The listing builds one solid part. Answer for the finished solid, in the listing's coordinates (mm). Face numbers are marked on the shaded views. Give positions to 0.01 mm unless a question says otherwise; leave off trailing zeros. Order: outer loops, then holes, each group sorted by start corner. A loop starts at its lowest first (then second) coordinate and runs counter-clockwise, first axis right, second up. Notation, with made-up numbers: (22, -17) - (26, -17) arc R24 ccw to (26, -1) - close; hole circle Ø2 at (23.5, 56). An arc over 180 degrees is marked (long way). Answer as a JSON object with one key per item and string values. Group by question number.
Q1. The mould has two halves that part along Y. Classify the marked faces 1 and 2: released by +Y, released by -Y, zero draft, split by the parting line, or undercut.
Q2. Consider line 1 (Y direction, x = 59.5, z = 9.5); line 2 (X direction, y = -17.5, z = 1.25); line 3 (Y direction, x = 11, z = -0.5). Determine where each line is inside the solid, lowest interval first.
Q3. A cutting plane is placed at C-C, the plane y = -31. Give the vertices of the cut face in (x, z), and give its area (3 significant figures).
Q4. Given pin 1 (2 mm diameter, centred on x = 16.5, y = -4, fed in from +Z); pin 2 (12 mm diameter, centred on x = 37, z = 12.5, fed in from +Y); pin 3 (9.5 mm diameter, centred on y = -13, z = 9, fed in from -X); pin 4 (10.5 mm diameter, centred on x = 26, z = 4, fed in from +Y), each flat-ended and moving along its own axis, determine where each tip first touches the part or whether it passes through.
Q5. A cutting plane is placed at A-A, the plane z = -1.25. Give the vertices of the cut face in (x, y), and give its area (3 significant figures).
Q6. A cutting plane is placed at B-B, the plane x = 45.5. Give the vertices of the cut face in (y, z).
from build123d import *

# Parameters (mm, degrees)
SKETCH1_W           = 52
SKETCH1_H           = 32
BOSS_EXTRUDE1_DEPTH = 3
SKETCH2_W           = 4
SKETCH2_H           = 32
BOSS_EXTRUDE2_DEPTH = 20
FILLET1_R           = 3
SKETCH4_R           = 1.725
CUT_EXTRUDE2_DEPTH  = 3
SKETCH6_W           = 20
SKETCH6_H           = 14
CUT_EXTRUDE3_DEPTH  = 3
SKETCH7_W           = 8.2
SKETCH7_H           = 5.8
SKETCH7_W_2         = 5.8
SKETCH7_H_2         = 3.4
BOSS_EXTRUDE4_DEPTH = 6
SKETCH10_R          = 4.9
SKETCH10_R_2        = 4
BOSS_EXTRUDE6_DEPTH = 10
SKETCH8_R           = 5.4
SKETCH8_R_2         = 4.25
BOSS_EXTRUDE5_DEPTH = 6
FILLET2_R           = 2
FILLET3_R           = 3
BOSS_EXTRUDE7_DEPTH = 48


with BuildPart() as part:
    # Sketch1 → Boss-Extrude1 (new body)
    with BuildSketch(Plane.XY):
        with Locations((26, -16)):
            Rectangle(SKETCH1_W, SKETCH1_H)
    extrude(amount=BOSS_EXTRUDE1_DEPTH)

    # Sketch2 → Boss-Extrude2 (add)
    with BuildSketch(Plane(origin=(0, 0, 2), x_dir=(-1, 0, 0), z_dir=(0, 0, -1))):
        with Locations((-50, -16)):
            Rectangle(SKETCH2_W, SKETCH2_H)
    extrude(amount=-BOSS_EXTRUDE2_DEPTH)

    # Fillet1
    fillet1_edges = [part.edges().sort_by_distance(p)[0] for p in [
        (50, -32, 22),
        (50, 0, 22),
    ]]
    fillet(fillet1_edges, radius=FILLET1_R)

    # Sketch4 → Cut-Extrude2 (cut)
    with BuildSketch(Plane.XY.offset(3)):
        with Locations((41.277695867, -8)):
            Circle(SKETCH4_R)
        with Locations((6.277695867, -8)):
            Circle(SKETCH4_R)
    extrude(amount=-CUT_EXTRUDE2_DEPTH, mode=Mode.SUBTRACT)

    # Sketch6 → Cut-Extrude3 (cut)
    with BuildSketch(Plane.XY.offset(3)):
        with Locations((23.277695867, -16)):
            Rectangle(SKETCH6_W, SKETCH6_H)
    extrude(amount=-CUT_EXTRUDE3_DEPTH, mode=Mode.SUBTRACT)

    # Sketch7 → Boss-Extrude4 (add)
    with BuildSketch(Plane(origin=(52, 0, 0), x_dir=(0, 0, -1), z_dir=(1, 0, 0))):
        with Locations((-9.5, -16)):
            Rectangle(SKETCH7_W, SKETCH7_H)
        with Locations((-9.5, -16)):
            Rectangle(SKETCH7_W_2, SKETCH7_H_2, mode=Mode.SUBTRACT)
    extrude(amount=BOSS_EXTRUDE4_DEPTH)

    # Sketch10 → Boss-Extrude6 (add)
    with BuildSketch(Plane(origin=(52, 0, 0), x_dir=(0, 0, -1), z_dir=(1, 0, 0))):
        with Locations(Location((-9.5, -16, 0), (0, 0, 146.796900802))):
            Circle(SKETCH10_R)
        with Locations(Location((-9.5, -16, 0), (0, 0, 133.531152167))):
            Circle(SKETCH10_R_2, mode=Mode.SUBTRACT)
    extrude(amount=BOSS_EXTRUDE6_DEPTH)

    # Sketch8 → Boss-Extrude5 (add)
    with BuildSketch(Plane(origin=(52, 0, 0), x_dir=(0, 0, -1), z_dir=(1, 0, 0))):
        with Locations(Location((-9.5, -16, 0), (0, 0, 270))):
            Circle(SKETCH8_R)
        with Locations((-9.5, -16)):
            Circle(SKETCH8_R_2, mode=Mode.SUBTRACT)
    extrude(amount=BOSS_EXTRUDE5_DEPTH)

    # Fillet2
    fillet2_edges = [part.edges().sort_by_distance(p)[0] for p in [
        (33.277695867, -9, 1.5),
        (33.277695867, -23, 1.5),
        (13.277695867, -23, 1.5),
        (13.277695867, -9, 1.5),
    ]]
    fillet(fillet2_edges, radius=FILLET2_R)

    # Fillet3
    # the kernel refuses this fillet: 3 mm, written as the material it adds along each edge
    with BuildSketch(Plane(origin=(52, -16, 9.5), x_dir=(0, -1, 0), z_dir=(0, 0, 1))) as fillet3_piece_1:
        with BuildLine():
            CenterArc((5.4 + FILLET3_R, FILLET3_R), FILLET3_R, 180, 90)
            Line((5.4, FILLET3_R), (5.4, 0))
            Line((5.4, 0), (5.4 + FILLET3_R, 0))
        make_face()
    revolve(axis=Axis((52, -16, 9.5), (1, 0, 0)))
    # the kernel refuses this fillet: 3 mm, written as the material it takes off along each edge
    with BuildSketch(Plane(origin=(58, -16, 9.5), x_dir=(0, -1, 0), z_dir=(0, 0, 1))) as fillet3_2_piece_1:
        with BuildLine():
            CenterArc((2.4, -1.658312395), FILLET3_R, 0, 33.557309762)
            Line((4.9, 0), (5.4, 0))
            Line((5.4, 0), (5.4, -1.658312395))
        make_face()
    revolve(axis=Axis((58, -16, 9.5), (1, 0, 0)), mode=Mode.SUBTRACT)

    # Sketch15 → Boss-Extrude7 (add)
    with BuildSketch(Plane.ZY):
        Polygon((-3.5, -2), (-3.5, 1.5), (-2, 1.5), (-2, 0), (0, 0), (0, -2), align=None)
        Polygon((-3.5, -33.5), (-2, -33.5), (-2, -32), (0, -32), (0, -30), (-3.5, -30), align=None)
    extrude(amount=-BOSS_EXTRUDE7_DEPTH)


solid = part.part
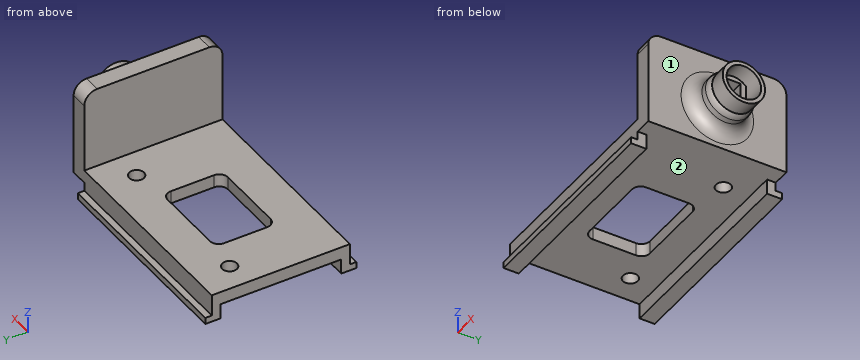
Reply:
{
 "1": {"face 1": "zero draft", "face 2": "undercut"},
 "2": {"line 1": "y = -20.9 to -20, -12 to -11.1", "line 2": "x = 0 to 13.28, 33.28 to 52", "line 3": "y = -32 to -30, -2 to 0"},
 "3": {"outline": "(0, -3.5) - (48, -3.5) - (48, 0) - (52, 0) - (52, 21.24) - (48, 21.24) - (48, 3) - (0, 3) - close", "area": "397 mm^2"},
 "4": {"pin 1": "stops at z = 3", "pin 2": "passes through", "pin 3": "stops at x = 48", "pin 4": "stops at y = 0"},
 "5": {"outline": "(0, -32) - (48, -32) - (48, -30) - (0, -30) - close; (0, -2) - (48, -2) - (48, 0) - (0, 0) - close", "area": "192 mm^2"},
 "6": {"outline": "(-33.5, -3.5) - (-30, -3.5) - (-30, 0) - (-2, 0) - (-2, -3.5) - (1.5, -3.5) - (1.5, -2) - (0, -2) - (0, 3) - (-32, 3) - (-32, -2) - (-33.5, -2) - close"}
}
